from build123d import *

# Parameters (mm, degrees)
SKETCH3_R                = 43.942
BOSS_EXTRUDE1_DEPTH      = 15.24
BOSS_EXTRUDE2_REACH      = 2331.885
BOSS_EXTRUDE2_END_RADIUS = 78.322932
SKETCH4_W                = 3.175
SKETCH4_H                = 203.2
CUT_EXTRUDE1_REACH       = 2322.063
FILLET1_R                = 2.54
CIRPATTERN1_COUNT        = 4
FILLET1_OF_CIRPATTERN1_R = 2.54


with BuildPart() as part:
    # Sketch2 → Revolve1 (revolve)
    with BuildSketch(Plane(origin=(0, 0, 0), x_dir=(0, 0, -1), z_dir=(1, 0, 0)), mode=Mode.PRIVATE) as revolve1_sk:
        with BuildLine():
            Line((254, 78.322932), (2289.4925, 78.322932))
            Line((2289.4925, 78.322932), (2289.4925, 0))
            Line((2289.4925, 0), (0, 0))
            add(Edge.make_bspline(
                [(254, 78.322932), (0, 78.322932), (0, 0)],
                knots=[4.71238898, 4.71238898, 4.71238898, 6.283185307, 6.283185307, 6.283185307], degree=2, weights=[1, 0.707106781, 1]))
        make_face()
    revolve(revolve1_sk.sketch.rotate(Axis((0, 0, -2289.4925), (0, 0, 1)), 90), axis=Axis((0, 0, -2289.4925), (0, 0, 1)))

    # Sketch3 → Boss-Extrude1 (add)
    with BuildSketch(Plane(origin=(0, 0, -2289.4925), x_dir=(-1, 0, 0), z_dir=(0, 0, -1))):
        with Locations(Location((0, 0, 0), (0, 0, 270))):
            Circle(SKETCH3_R)
    extrude(amount=BOSS_EXTRUDE1_DEPTH)

    # Boss-Extrude2: up to this cylinder (the profile starts outside it)
    boss_extrude2_end = Plane(origin=(0, 0, -2184.7175), z_dir=(0, 0, -1)) * Cylinder(BOSS_EXTRUDE2_END_RADIUS, 4821.415864, mode=Mode.PRIVATE)
    # Sketch4 → Boss-Extrude2 (add, up to the surface)
    with BuildSketch(Plane(origin=(0, 254, 0), x_dir=(1, 0, 0), z_dir=(0, 1, 0)), mode=Mode.PRIVATE) as boss_extrude2_sk1:
        with Locations((0, 2184.7175)):
            Rectangle(SKETCH4_W, SKETCH4_H)
    boss_extrude2_tool1 = extrude(boss_extrude2_sk1.sketch, amount=-BOSS_EXTRUDE2_REACH, mode=Mode.PRIVATE) - boss_extrude2_end
    boss_extrude2 = boss_extrude2_tool1.solids().sort_by_distance((0, 254, -2184.7175))[0]
    add(boss_extrude2)

    # Sketch5 → Cut-Extrude1 (cut, up to next)
    with BuildSketch(Plane.ZY.offset(1.5875), mode=Mode.PRIVATE) as cut_extrude1_sk1:
        Polygon((-2286.3175, 224.356842107), (-2184.7175, 224.356842107), (-2083.1175, 78.306842107), (-2083.1175, 254), (-2286.3175, 254), align=None)
    cut_extrude1_tool1 = extrude(cut_extrude1_sk1.sketch, amount=-CUT_EXTRUDE1_REACH, mode=Mode.PRIVATE) & part.part
    cut_extrude1 = cut_extrude1_tool1.solids().sort_by_distance((-1.5875, 204.128915, -2147.334252))[0]
    add(cut_extrude1, mode=Mode.SUBTRACT)

    # Fillet1
    # the kernel refuses this fillet: 2.54 mm, written as the material it adds along each edge
    with BuildSketch(Plane(origin=(-1.5875, 78.306842107, -2076.990797857), x_dir=(-0.9993639751499004, -0.03566013422001241, 0), z_dir=(0, 0, -1))) as fillet1_piece_1_section:
        with BuildLine():
            CenterArc((2.450992889, 2.539698904), FILLET1_R, 182.043608468, 87.074170625)
            Line((-0.087391608, 2.449122163), (0, 0))
            ThreePointArc((0, 0), (1.205942189, 0.009284527), (2.411884379, 0))
        make_face()
    fillet1_piece_1 = extrude(amount=209.326702143, mode=Mode.PRIVATE)
    fillet1_piece_1 = split(fillet1_piece_1, bisect_by=Plane(origin=(-3.095055571, 78.248638535, -2083.077010558), z_dir=(0, -0.5710644881985995, -0.8209052017854874)), keep=Keep.TOP, mode=Mode.PRIVATE)
    add(fillet1_piece_1)
    with BuildSketch(Plane(origin=(1.5875, 78.306842107, -2076.990797857), x_dir=(0.9993639751499004, -0.035660134220013434, 0), z_dir=(0, 0, -1))) as fillet1_piece_2_section:
        with BuildLine():
            CenterArc((2.450992889, -2.539698904), FILLET1_R, 90.882220907, 87.074170625)
            Line((-0.087391608, -2.449122163), (0, 0))
            ThreePointArc((0, 0), (1.205942189, -0.009284527), (2.411884379, 0))
        make_face()
    fillet1_piece_2 = extrude(amount=209.326702143, mode=Mode.PRIVATE)
    fillet1_piece_2 = split(fillet1_piece_2, bisect_by=Plane(origin=(3.095055571, 78.248638535, -2083.077010558), z_dir=(0, -0.5710644881985995, -0.8209052017854874)), keep=Keep.TOP, mode=Mode.PRIVATE)
    add(fillet1_piece_2)

    # CirPattern1: Boss-Extrude2, Cut-Extrude1 ×4 about axis
    cirpattern1_axis = Axis((0, 0, 0), (0, 0, 1))
    add([boss_extrude2.rotate(cirpattern1_axis, i * 360 / CIRPATTERN1_COUNT) for i in range(1, CIRPATTERN1_COUNT)])
    add([cut_extrude1.rotate(cirpattern1_axis, i * 360 / CIRPATTERN1_COUNT) for i in range(1, CIRPATTERN1_COUNT)], mode=Mode.SUBTRACT)

    # Fillet1 of CirPattern1
    # the kernel refuses this fillet: 2.54 mm, written as the material it adds along each edge
    with BuildSketch(Plane(origin=(-78.306842107, -1.5875, -2076.990797857), x_dir=(0.035660134220018486, -0.9993639751499002, 0), z_dir=(0, 0, -1))) as fillet1_of_cirpattern1_piece_1_section:
        with BuildLine():
            CenterArc((2.450992889, 2.539698904), FILLET1_OF_CIRPATTERN1_R, 182.043608468, 87.074170625)
            Line((-0.087391608, 2.449122163), (0, 0))
            ThreePointArc((0, 0), (1.205942189, 0.009284527), (2.411884379, 0))
        make_face()
    fillet1_of_cirpattern1_piece_1 = extrude(amount=209.326702143, mode=Mode.PRIVATE)
    fillet1_of_cirpattern1_piece_1 = split(fillet1_of_cirpattern1_piece_1, bisect_by=Plane(origin=(-78.248638535, -3.095055571, -2083.077010558), z_dir=(0.5710644881985995, 0, -0.8209052017854874)), keep=Keep.TOP, mode=Mode.PRIVATE)
    add(fillet1_of_cirpattern1_piece_1)
    with BuildSketch(Plane(origin=(-78.306842107, 1.5875, -2076.990797857), x_dir=(0.03566013422001241, 0.9993639751499004, 0), z_dir=(0, 0, -1))) as fillet1_of_cirpattern1_piece_2_section:
        with BuildLine():
            CenterArc((2.450992889, -2.539698904), FILLET1_OF_CIRPATTERN1_R, 90.882220907, 87.074170625)
            Line((-0.087391608, -2.449122163), (0, 0))
            ThreePointArc((0, 0), (1.205942189, -0.009284527), (2.411884379, 0))
        make_face()
    fillet1_of_cirpattern1_piece_2 = extrude(amount=209.326702143, mode=Mode.PRIVATE)
    fillet1_of_cirpattern1_piece_2 = split(fillet1_of_cirpattern1_piece_2, bisect_by=Plane(origin=(-78.248638535, 3.095055571, -2083.077010558), z_dir=(0.5710644881985995, 0, -0.8209052017854874)), keep=Keep.TOP, mode=Mode.PRIVATE)
    add(fillet1_of_cirpattern1_piece_2)
    with BuildSketch(Plane(origin=(1.5875, -78.306842107, -2076.990797857), x_dir=(0.9993639751499002, 0.035660134220018555, 0), z_dir=(0, 0, -1))) as fillet1_of_cirpattern1_piece_3_section:
        with BuildLine():
            CenterArc((2.450992889, 2.539698904), FILLET1_OF_CIRPATTERN1_R, 182.043608468, 87.074170625)
            Line((-0.087391608, 2.449122163), (0, 0))
            ThreePointArc((0, 0), (1.205942189, 0.009284527), (2.411884379, 0))
        make_face()
    fillet1_of_cirpattern1_piece_3 = extrude(amount=209.326702143, mode=Mode.PRIVATE)
    fillet1_of_cirpattern1_piece_3 = split(fillet1_of_cirpattern1_piece_3, bisect_by=Plane(origin=(3.095055571, -78.248638535, -2083.077010558), z_dir=(0, 0.5710644881985995, -0.8209052017854874)), keep=Keep.TOP, mode=Mode.PRIVATE)
    add(fillet1_of_cirpattern1_piece_3)
    with BuildSketch(Plane(origin=(-1.5875, -78.306842107, -2076.990797857), x_dir=(-0.9993639751499004, 0.03566013422001239, 0), z_dir=(0, 0, -1))) as fillet1_of_cirpattern1_piece_4_section:
        with BuildLine():
            CenterArc((2.450992889, -2.539698904), FILLET1_OF_CIRPATTERN1_R, 90.882220907, 87.074170625)
            Line((-0.087391608, -2.449122163), (0, 0))
            ThreePointArc((0, 0), (1.205942189, -0.009284527), (2.411884379, 0))
        make_face()
    fillet1_of_cirpattern1_piece_4 = extrude(amount=209.326702143, mode=Mode.PRIVATE)
    fillet1_of_cirpattern1_piece_4 = split(fillet1_of_cirpattern1_piece_4, bisect_by=Plane(origin=(-3.095055571, -78.248638535, -2083.077010558), z_dir=(0, 0.5710644881985995, -0.8209052017854874)), keep=Keep.TOP, mode=Mode.PRIVATE)
    add(fillet1_of_cirpattern1_piece_4)
    with BuildSketch(Plane(origin=(78.306842107, 1.5875, -2076.990797857), x_dir=(-0.03566013422001241, 0.9993639751499004, 0), z_dir=(0, 0, -1))) as fillet1_of_cirpattern1_piece_5_section:
        with BuildLine():
            CenterArc((2.450992889, 2.539698904), FILLET1_OF_CIRPATTERN1_R, 182.043608468, 87.074170625)
            Line((-0.087391608, 2.449122163), (0, 0))
            ThreePointArc((0, 0), (1.205942189, 0.009284527), (2.411884379, 0))
        make_face()
    fillet1_of_cirpattern1_piece_5 = extrude(amount=209.326702143, mode=Mode.PRIVATE)
    fillet1_of_cirpattern1_piece_5 = split(fillet1_of_cirpattern1_piece_5, bisect_by=Plane(origin=(78.248638535, 3.095055571, -2083.077010558), z_dir=(-0.5710644881985995, 0, -0.8209052017854874)), keep=Keep.TOP, mode=Mode.PRIVATE)
    add(fillet1_of_cirpattern1_piece_5)
    with BuildSketch(Plane(origin=(78.306842107, -1.5875, -2076.990797857), x_dir=(-0.03566013422001239, -0.9993639751499004, 0), z_dir=(0, 0, -1))) as fillet1_of_cirpattern1_piece_6_section:
        with BuildLine():
            CenterArc((2.450992889, -2.539698904), FILLET1_OF_CIRPATTERN1_R, 90.882220907, 87.074170625)
            Line((-0.087391608, -2.449122163), (0, 0))
            ThreePointArc((0, 0), (1.205942189, -0.009284527), (2.411884379, 0))
        make_face()
    fillet1_of_cirpattern1_piece_6 = extrude(amount=209.326702143, mode=Mode.PRIVATE)
    fillet1_of_cirpattern1_piece_6 = split(fillet1_of_cirpattern1_piece_6, bisect_by=Plane(origin=(78.248638535, -3.095055571, -2083.077010558), z_dir=(-0.5710644881985995, 0, -0.8209052017854874)), keep=Keep.TOP, mode=Mode.PRIVATE)
    add(fillet1_of_cirpattern1_piece_6)


solid = part.part
Source: CAD feature listing. Evaluate the final solid. Frame: model axes, mm. A direction names the side the tool comes from. Coordinates: 2 decimals unless noted, no trailing zeros. Loops run counter-clockwise (first coordinate to the right, second up) from the corner with the lowest first, then second, coordinate; pieces in that order, holes last. Notation, with made-up numbers: (46, 57.5) - (95, 57.5) arc R34 cw to (95, 90.5) - close; hole circle Ø5 at (-11.75, 2). An arc over 180 degrees is marked (long way). One line per item, written item: value. Start each with the question number.
1. Ray query, L1, parallel to Y at x = 4.5, z = -1815.5; L2, parallel to Y at x = 144, z = -2170.5; L3, parallel to X at y = -59, z = -1287.5. Return the intervals inside material, ascending.
2. Contact query for flat-ended pins moving along their axis: P1, Ø9, axis at x = 0.5, y = 140.5, coming from the -Z side; P2, Ø8, axis at y = -4.5, z = -1020.5, coming from the +X side; P3, Ø12, axis at x = 68, z = -1513.5, coming from the +Y side. Output: stop coordinate, or through.
3. Section A-A (z = -641). Return the cut outline in (x, y), and give its area (3 significant figures).
4. Set-up query: faces 1 (the flat face through (-34, 34, -2289.492)), 2 (the flat face through (-1.588, 154, -2207)), 3 (the flat face through (154, -1.588, -2207)). Return all of +Z, -Z, +X, -X, +Y, -Y with unobstructed straight access to the full face (end or side cutting, diameter ignored); none if empty.
Verdict:
1. L1: y = -78.19 to 78.19
1. L2: y = -1.59 to 1.59
1. L3: x = -51.51 to 51.51
2. P1: stops at z = -2286.32
2. P2: stops at x = 78.32
2. P3: stops at y = 47.86
3. outline: circle Ø156.65 at (0, 0)
3. area: 19,300 mm2
4. face 1: -Z
4. face 2: +Z, -Z, -X, +Y
4. face 3: +Z, -Z, +X, -Y
